```python
from build123d import *

# Parameters (mm, degrees)
F1_DEPTH = 30
F3_DEPTH = 3
F5_DEPTH = 3
F6_R     = 4
F7_R     = 3
F8_R     = 5.1


with BuildPart() as f1:
    # F0 (on Front) → F1 (new body)
    with BuildSketch(Plane.XZ):
        with BuildLine():
            Line((-23.262718, 0), (0, 0))
            Line((0, 0), (23.262718, 0))
            Line((23.262718, 0), (23.262718, 11.85973))
            Line((23.262718, 11.85973), (34.820285, 33.596352))
            Line((34.820285, 33.596352), (30.695623, 33.596352))
            ThreePointArc((30.695623, 33.596352), (0, 9.169452), (-30.695623, 33.596352))
            Line((-30.695623, 33.596352), (-34.820285, 33.596352))
            Line((-34.820285, 33.596352), (-23.262718, 11.85973))
            Line((-23.262718, 11.85973), (-23.262718, 0))
        make_face()
    extrude(amount=F1_DEPTH)

    # F2 (on face) → F3 (join)
    with BuildSketch(Plane.XZ.offset(30)):
        with BuildLine():
            ThreePointArc((34.820285, 33.596352), (0, 22.458891), (-34.820285, 33.596352))
            Line((-34.820285, 33.596352), (-23.262718, 11.85973))
            Line((-23.262718, 11.85973), (-23.262718, 0))
            Line((-23.262718, 0), (23.262718, 0))
            Line((23.262718, 0), (23.262718, 11.85973))
            Line((23.262718, 11.85973), (34.820285, 33.596352))
        make_face()
    extrude(amount=F3_DEPTH)

    # F4 (on face) → F5 (join)
    with BuildSketch(Plane(origin=(0, 0, 0), x_dir=(-1, 0, 0), z_dir=(0, 1, 0))):
        with BuildLine():
            ThreePointArc((34.820285, 33.596352), (0, 22.458891), (-34.820285, 33.596352))
            Line((-34.820285, 33.596352), (-23.262718, 11.85973))
            Line((-23.262718, 11.85973), (-23.262718, 0))
            Line((-23.262718, 0), (23.262718, 0))
            Line((23.262718, 0), (23.262718, 11.85973))
            Line((23.262718, 11.85973), (34.820285, 33.596352))
        make_face()
    extrude(amount=F5_DEPTH)

    # F6
    f6_edges = [f1.edges().sort_by_distance(p)[0] for p in [
        (30.695623, -15, 33.596352),
        (-30.695623, -15, 33.596352),
    ]]
    fillet(f6_edges, radius=F6_R)

    # F7
    f7_edges = [f1.edges().sort_by_distance(p)[0] for p in [
        (23.262718, -15, 0),
        (0, 3, 0),
        (-23.262718, -15, 0),
        (0, -33, 0),
    ]]
    fillet(f7_edges, radius=F7_R)

    # F8
    f8_edges = [f1.edges().sort_by_distance(p)[0] for p in [
        (-23.262718, -15, 11.85973),
        (23.262718, -15, 11.85973),
    ]]
    fillet(f8_edges, radius=F8_R)


solid = f1.part
```
Part model, mm, in its own coordinate system. A direction names the side the tool comes from. Give positions to 0.01 mm unless a question says otherwise; leave off trailing zeros. Order: outer loops, then holes, each group sorted by start corner. A loop starts at its lowest first (then second) coordinate and runs counter-clockwise, first axis right, second up. Notation, with made-up numbers: M 38.5,-4.5 L 66.5,-4.5 A19 cw 66.5,5.5 Z; hole C 0,68 d6. An arc over 180 degrees is marked long. Use a Markdown table: item, result. Add a question column.
(1) Saw through at D-D, the plane x = -14. Give the cut face in (y, z).
(2) Saw through at B-B, the plane z = 19. Give the cut face in (x, y).
(3) Drop flat-ended pins along their axis: P1, Ø4, axis at y = -21, z = 8, coming from the +X side; P2, Ø10, axis at y = -3.5, z = 17, coming from the +X side; P3, Ø5, axis at y = -11.5, z = 4, coming from the -X side. Give the stop position or say it passes through.
(4) Probe line 1 along Y through (x, z) = (6, 13); line 2 along X through (y, z) = (-14, 4); line 3 along X through (y, z) = (-9.5, 12). List the from-to ranges inside material, lowest first. Write a range as [from, to].
(5) 3-axis set-ups, long thin cutter, end or side, ignore diameter. For faces 4 (the face through (23.263, -15, 7)), 5 (the face through (-23.263, -15, 7)), 6 (the face through (0.553, -14.79, 9.174)), 7 (the face through (-31.354, -15.21, 32.815)), 8 (the face through (-0.52, 1.48, 22.46)): which of +Z, -Z, +X, -X, +Y, -Y reach the whole face in a straight line?
(6) Saw through at C-C, the plane z = 26. Give the cut face in (x, y), and give its area (3 significant figures).
(7) Saw through at A-A, the plane y = -26. Give the cut face in (x, z), and give its area (3 significant figures).
(8) Mould opens along Y. For faces 1 (the face through (0, -30, 18)), 2 (the face through (0, 3, 15)), 3 (the face through (0, -15, 0)) say: +Y half, -Y half, draft (parallel to the pull), parting line (faces both ways), or undercut.
Answer key:
| question | item | result |
|---|---|---|
| 1 | outline | M -33,3 A3 ccw -30,0 L 0,0 A3 ccw 3,3 L 3,24.12 L 0,24.12 L 0,12.45 L -30,12.45 L -30,24.12 L -33,24.12 Z |
| 2 | outline | M -27.06,-33 L 27.06,-33 L 27.06,3 L -27.06,3 Z; hole M -22.86,-30 L 22.86,-30 L 22.86,0 L -22.86,0 Z |
| 3 | P1 | x = 23.26 |
| 3 | P2 | x = 28.65 |
| 3 | P3 | x = -23.26 |
| 4 | line 1 | [-33, -30], [0, 3] |
| 4 | line 2 | [-23.26, 23.26] |
| 4 | line 3 | [-23.46, -13.05], [13.05, 23.46] |
| 5 | face 4 | -Z, +X, +Y, -Y |
| 5 | face 5 | -Z, -X, +Y, -Y |
| 5 | face 6 | +Z |
| 5 | face 7 | +Z, +Y, -Y |
| 5 | face 8 | +Z, +Y |
| 6 | outline | M -30.78,-33 L -20.31,-33 L -20.31,-30 L -27.88,-30 L -27.88,0 L -20.31,0 L -20.31,3 L -30.78,3 Z; M 20.31,-33 L 30.78,-33 L 30.78,3 L 20.31,3 L 20.31,0 L 27.88,0 L 27.88,-30 L 20.31,-30 Z |
| 6 | area | 300 mm^2 |
| 7 | outline | M -34.82,33.6 L -23.86,12.98 A5.1 cw -23.26,10.59 L -23.26,3 A3 ccw -20.26,0 L 20.26,0 A3 ccw 23.26,3 L 23.26,10.59 A5.1 cw 23.86,12.98 L 34.82,33.6 L 33.73,33.6 A4 ccw 29.93,30.84 A31.5 cw -29.93,30.84 A4 ccw -33.73,33.6 Z |
| 7 | area | 691 mm^2 |
| 8 | face 1 | undercut |
| 8 | face 2 | +Y half |
| 8 | face 3 | draft |
